Geometry: final body of the model. Coordinates: model frame, mm. Give positions to 0.01 mm unless a question says otherwise; leave off trailing zeros. Order: outer loops, then holes, each group sorted by start corner. A loop starts at its lowest first (then second) coordinate and runs counter-clockwise, first axis right, second up. Notation, with made-up numbers: (56, 81.25) -> (79, 81.25) arc R24 cw to (79, 118.25) -> close; hole circle Ø5 at (9, 43). An arc over 180 degrees is marked (long way). Write item = value, one per line.
Autodesk Inventor part; units mm, degrees
ref_plane "YZ Plane" through (0, 0, 0) normal (1, 0, 0) x (0, 1, 0)
ref_plane "XZ Plane" through (0, 0, 0) normal (0, 1, 0) x (-1, 0, 0)
ref_plane "XY Plane" through (0, 0, 0) normal (0, 0, 1) x (1, 0, 0)
sketch "Sketch1" plane through (0, 0, 0) normal (0, 0, 1) x (1, 0, 0)
  circle A0 centre (0, 0) radius 3
  dimension "d0" = 6
extrude "Extrusion1" add sketch "Sketch1" along normal blind 460
chamfer "Chamfer1" distance 0.5 angle 45 1 edges at (-3, 0, 0)
chamfer "Chamfer2" distance 0.5 angle 45 1 edges at (-3, 0, 460)
properties part number "6mmx460mmSmoothRod"
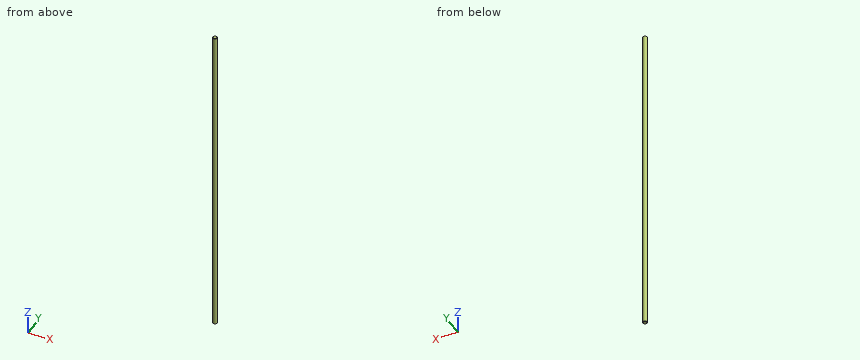
1) Line query: line 1 (Y direction, x = -0.5, z = 189); line 2 (X direction, y = -0.1, z = 27.5); line 3 (X direction, y = -1.6, z = 194). Output: solid intervals per line, ascending. Write a range as from..to.
Check sheet entries:
line_1 = -2.96..2.96
line_2 = -3..3
line_3 = -2.54..2.54
2) Section query A-A (z = 313). Output: boundary loops of the cut face in (x, y), plus the area to 3 significant figures.
Check sheet entries:
outline = circle Ø6 at (0, 0)
area = 28.3 mm²
3) First-contact query: P1, Ø1, axis at y = -2, z = 165, coming from the +X side; P2, Ø1, axis at x = -1.5, z = 105.5, coming from the -Y side; P3, Ø1.5, axis at x = 1, z = 64.5, coming from the +Y side. Flat tips, straight axial feed; report the tip coordinate or a pass-through.
Check sheet entries:
P1 = 2.6
P2 = -2.83
P3 = 2.99
